Can you work these out from the model? Positions are in its coordinate system, mm. A direction names the side the tool comes from. Give positions to 0.01 mm unless a question says otherwise; leave off trailing zeros. Order: outer loops, then holes, each group sorted by start corner. A loop starts at its lowest first (then second) coordinate and runs counter-clockwise, first axis right, second up. Notation, with made-up numbers: (4, -22.75) - (11, -22.75) arc R19 cw to (11, 9.25) - close; hole circle Ø10 at (-19, -26). An arc over 180 degrees is marked (long way). Answer as CSV lines item,"result".
Autodesk Inventor part; units mm, degrees
ref_plane "YZ Plane" through (0, 0, 0) normal (1, 0, 0) x (0, 1, 0)
ref_plane "XZ Plane" through (0, 0, 0) normal (0, 1, 0) x (-1, 0, 0)
ref_plane "XY Plane" through (0, 0, 0) normal (0, 0, 1) x (1, 0, 0)
sketch "Skizze1" plane through (0, 0, 0) normal (0, 0, 1) x (1, 0, 0)
  circle A0 centre (7.5, 13) radius 1.7
  circle A1 centre (7.5, 37) radius 1.7
  arc A2 (15.5, 37.6806) -> (13.0863, 41.3526) centre (11.5, 37.6806) ccw
  arc A3 (13.0863, 41.3526) -> (2.4137, 41.3526) centre (7.75, 29) ccw
  arc A4 (2.4137, 41.3526) -> (0, 37.6806) centre (4, 37.6806) ccw
  line L0 (0, 2.3194) -> (0, 37.6806)
  arc A5 (0, 2.3194) -> (2.4137, -1.3526) centre (4, 2.3194) ccw
  arc A6 (2.4137, -1.3526) -> (13.0863, -1.3526) centre (7.75, 11) ccw
  arc A7 (13.0863, -1.3526) -> (15.5, 2.3194) centre (11.5, 2.3194) ccw
  line L1 (15.5, 2.3194) -> (15.5, 37.6806)
  point P0 (0, 0)
extrude "Extrusion1" add sketch "Skizze1" along normal blind 5
sketch "Skizze2" plane through (0, 0, 5) normal (0, 0, 1) x (1, 0, 0)
  arc A0 (2.4137, -1.3526) -> (13.0863, -1.3526) centre (7.75, 11) ccw
  arc A1 (13.0863, -1.3526) -> (15.5, 2.3194) centre (11.5, 2.3194) ccw
  line L0 (15.5, 2.3194) -> (15.5, 37.6806)
  arc A2 (15.5, 37.6806) -> (13.0863, 41.3526) centre (11.5, 37.6806) ccw
  arc A3 (13.0863, 41.3526) -> (2.4137, 41.3526) centre (7.75, 29) ccw
  arc A4 (2.4137, 41.3526) -> (0, 37.6806) centre (4, 37.6806) ccw
  line L1 (0, 37.6806) -> (0, 2.3194)
  arc A5 (0, 2.3194) -> (2.4137, -1.3526) centre (4, 2.3194) ccw
  circle A6 centre (7.5, 37) radius 1.7
  circle A7 centre (7.5, 13) radius 1.7
  line L2 (7.75, 20) -> (7.75, 20)
  line L3 (7.75, 20) -> (7.75, -2.4559)
  line L4 (7.75, -2.4559) -> (7.75, -2.4559)
  line L5 (7.75, -2.4559) -> (7.75, 20)
  point P0 (0, 0)
  point P1 (7.75, -2.4559)
  dimension "d2" = 44.9119
  dimension "d3" = 15.5
  dimension "d4" = 22.456
  dimension "d5" = 0
hole "Bohrung1" at (7.75, 20, 5) direction (0, 0, -1) diameter 6.05 depth 3.1
sketch "Skizze4" plane through (0, 0, 5) normal (0, 0, 1) x (1, 0, 0)
  circle A0 centre (7.5, 4.722) radius 1.9913
  point P0 (0, 0)
hole "Bohrung2" at (7.5, 4.722, 5) direction (0, 0, -1) diameter 3.3 end through all counterbore diameter 5.8 counterbore depth 2
move faces "Verschieben1" translate (0, 0, 1) faces at (13.3835, 17.8023, 0)
sketch "Skizze6" plane through (7.75, 11, 1) normal (0, 0, -1) x (-1, 0, 0)
  circle A0 centre (-5.37, 26.9384) radius 1
  circle A1 centre (5.81, 25.1971) radius 1
  circle A2 centre (5.81, 25.1971) radius 1.2
  circle A3 centre (-5.37, 26.9384) radius 1.2
  circle A4 centre (5.87, 26.9384) radius 1
  circle A5 centre (-5.37, 26.9384) radius 1
  circle A6 centre (5.87, 26.9384) radius 1.2
  arc A7 (4.9199, 26.9621) -> (4.4911, 27.5261) centre (5.45, 27.81) ccw
  circle A8 centre (-5.37, 26.9384) radius 1
  circle A9 centre (5.37, -8.778) radius 1
  circle A10 centre (-5.37, -8.778) radius 1
  circle A11 centre (5.45, 27.81) radius 1.2
  circle A12 centre (-5.37, -8.778) radius 1.2
  circle A13 centre (5.37, -8.778) radius 1.2
  point P0 (7.75, -11)
  dimension "d37" = 2.4
  dimension "d38" = 2.4
  dimension "d44" = 2.4
  dimension "d45" = 2.4
  dimension "d46" = 2.4
  dimension "d47" = 2.4
extrude "Extrusion4" cut sketch "Skizze6" against normal blind 3 contours A0 | A11 A6 | A6 A7 A4 A11 | A11 A4 A7 A6 | A4 A11 | A3 | A9 | A10 | A12 | A13
chamfer "Fase1" distance 0.6 angle 45 4 edges at (14.32, 37.9384, 4) (3.5, 38.81, 4) (3.58, 2.222, 4) (14.32, 2.222, 4)
equation "\"d4\" = 0.5 * d2"
equation "\"d37\" = d38"
equation "\"d44\" = d38"
equation "\"d45\" = d38"
equation "\"d46\" = d38"
equation "\"d47\" = d38"
properties part number "Front-Idlers_Housing-Cover"
1) I want a section at C-C on y = 20. Write out the boundary of the cut face in (x, z) (3 decimals).
Answer block:
outline,"(0, 1) - (15.5, 1) - (15.5, 5) - (10.775, 5) - (10.775, 1.9) - (4.725, 1.9) - (4.725, 5) - (0, 5) - close"
2) I'm going to push flat-ended pins straight in: P1, Ø2, axis at x = 2.38, y = 2.222, coming from the -Z side; P2, Ø3, axis at x = 8.5, y = 5, coming from the +Z side; P3, Ø2, axis at x = 7.5, y = 4.722, coming from the -Z side; P4, Ø1, axis at x = 13, z = 4, coming from the +Y side. Where does each tip first touch, or does it pass through?
Answer block:
P1,"z = 3.6"
P2,"z = 3"
P3,"through"
P4,"y = 41.59"
3) I want a section at B-B on x = 7. Write out the boundary of the cut face in (y, z).
Answer block:
outline,"(-2.44, 1) - (3.15, 1) - (3.15, 3) - (1.87, 3) - (1.87, 5) - (-2.44, 5) - close; (6.29, 1) - (11.38, 1) - (11.38, 5) - (7.58, 5) - (7.58, 3) - (6.29, 3) - close; (14.62, 1) - (35.38, 1) - (35.38, 5) - (22.93, 5) - (22.93, 1.9) - (17.07, 1.9) - (17.07, 5) - (14.62, 5) - close; (38.62, 1) - (42.44, 1) - (42.44, 5) - (38.62, 5) - close"
4) I want a section at A-A on y = 14. Write out the boundary of the cut face in (x, z), plus the area to 3 significant figures.
Answer block:
outline,"(0, 1) - (6.13, 1) - (6.13, 5) - (0, 5) - close; (8.87, 1) - (15.5, 1) - (15.5, 5) - (8.87, 5) - close"
area,"51.0 mm2"
5) If we mould it in two halves opening along X, with no side actions, what happens to faces 1 (the cylindrical face through (14.86, 0.15, 2.97)), 2 (the cylindrical face through (0.64, 39.85, 2.97)), 3 (the flat face through (2, 2, 4))? For each: +X half, -X half, draft (parallel to the pull), parting line (faces both ways), or undercut.
Answer block:
face 1,"+X half"
face 2,"-X half"
face 3,"undercut"
6) I need wall thicknesses on line 1 along X through (y, z) = (20, 4.05) (3 decimals); line 2 along Y through (x, z) = (13.12, 2); line 3 along Y through (x, z) = (7.5, 1.65). Which ranges of each line are inside material? Lowest first, please. Write a range as [from, to].
Answer block:
line 1,"[0, 4.725], [10.775, 15.5]"
line 2,"[-1.34, 1.02], [3.42, 36.74], [39.14, 41.34]"
line 3,"[-2.45, 3.07], [6.37, 11.3], [14.7, 35.3], [38.7, 42.45]"
7) I want a section at D-D on y = 4. Write out the boundary of the cut face in (x, z), plus the area to 3 significant figures.
Answer block:
outline,"(0, 1) - (6.02, 1) - (6.02, 3) - (4.69, 3) - (4.69, 5) - (0, 5) - close; (8.98, 1) - (15.5, 1) - (15.5, 5) - (10.31, 5) - (10.31, 3) - (8.98, 3) - close"
area,"44.8 mm2"
8) Which directions (+Z, -Z, +X, -X, +Y, -Y) give clear straight access to the entire face, cutting with the end or side of a thin tool? Please do faces 4 (the flat face through (2, 39, 4)), 5 (the cylindrical face through (7.13, 38.66, 2.97)), 6 (the cylindrical face through (9.59, 22.4, 3.43)).
Answer block:
face 4,"-Z"
face 5,"+Z, -Z"
face 6,"+Z"
